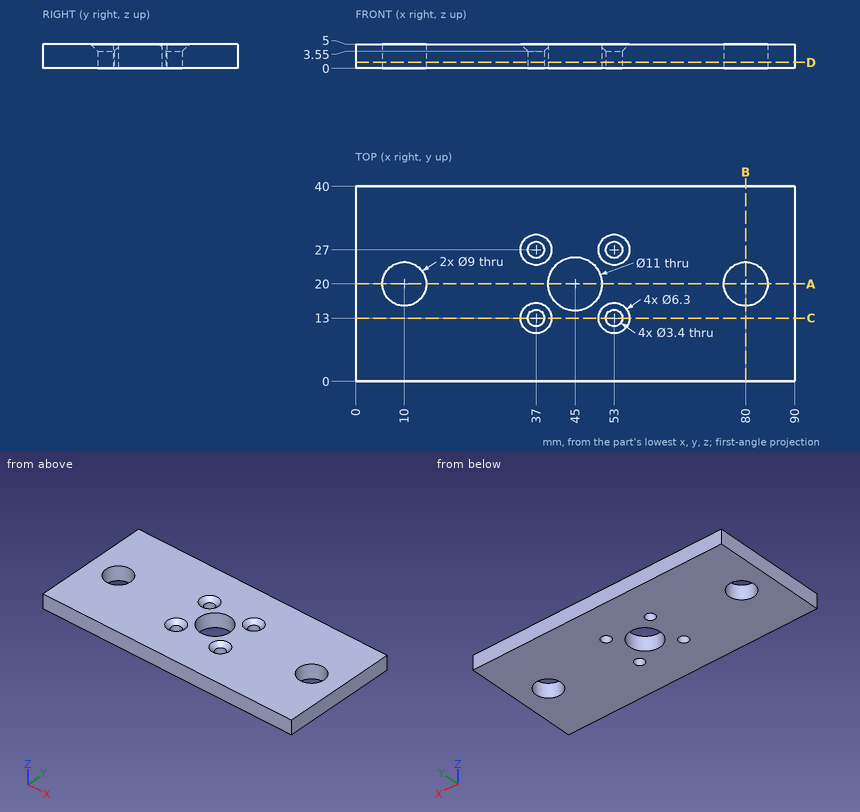
Check sheet for the drawn part. Datum: minimum x, y, z corner. Units: mm. Round coordinates to 2 decimals unless told otherwise and drop trailing zeros. Loops run counter-clockwise (first coordinate to the right, second up) from the corner with the lowest first, then second, coordinate; pieces in that order, holes last.
Item 1: Thickness scan on line 1 (X direction, y = 20, z = 2.35); line 2 (Y direction, x = 37, z = 2.4); line 3 (X direction, y = 13, z = 1.6). Record the ranges inside material, lowest first.
Item 2: Gauge pin test, flat ends, axial feed: pin 1 (2 mm diameter, centred on x = 53, y = 27, fed in from +Z); pin 2 (5 mm diameter, centred on x = 14, y = 19, fed in from +Z). Record the tip position at first contact, or that the pin passes through.
Item 3: Cross-section at B-B on x = 80. Record the boundary of the cut face in (y, z).
Item 4: Cross-section at A-A on y = 20. Record the boundary of the cut face in (x, z), then the cut area to 3 significant figures.
Item 5: Cross-section at D-D on z = 1.25. Record the boundary of the cut face in (x, y), then the cut area to 3 significant figures.
Item 6: Cross-section at C-C on y = 13. Record the boundary of the cut face in (x, z).
Answer sheet:
1. line 1: x = 0 to 5.5, 14.5 to 39.5, 50.5 to 75.5, 84.5 to 90
1. line 2: y = 0 to 11.3, 14.7 to 25.3, 28.7 to 40
1. line 3: x = 0 to 35.3, 38.7 to 51.3, 54.7 to 90
2. pin 1: passes through
2. pin 2: stops at z = 5
3. outline: (0, 0) - (15.5, 0) - (15.5, 5) - (0, 5) - close; (24.5, 0) - (40, 0) - (40, 5) - (24.5, 5) - close
4. outline: (0, 0) - (5.5, 0) - (5.5, 5) - (0, 5) - close; (14.5, 0) - (39.5, 0) - (39.5, 5) - (14.5, 5) - close; (50.5, 0) - (75.5, 0) - (75.5, 5) - (50.5, 5) - close; (84.5, 0) - (90, 0) - (90, 5) - (84.5, 5) - close
4. area: 305 mm2
5. outline: (0, 0) - (90, 0) - (90, 40) - (0, 40) - close; hole circle Ø9 at (10, 20); hole circle Ø3.4 at (37, 13); hole circle Ø3.4 at (37, 27); hole circle Ø11 at (45, 20); hole circle Ø3.4 at (53, 13); hole circle Ø3.4 at (53, 27); hole circle Ø9 at (80, 20)
5. area: 3,340 mm2
6. outline: (0, 0) - (35.3, 0) - (35.3, 3.55) - (33.85, 5) - (0, 5) - close; (38.7, 0) - (51.3, 0) - (51.3, 3.55) - (49.85, 5) - (40.15, 5) - (38.7, 3.55) - close; (54.7, 0) - (90, 0) - (90, 5) - (56.15, 5) - (54.7, 3.55) - close
